from build123d import *

# Parameters (mm, degrees)
SKETCH1_R           = 20
SKETCH1_R_2         = 2.5
BOSS_EXTRUDE1_DEPTH = 10
CUT_EXTRUDE1_DEPTH  = 30
FILLET1_R           = 6
CUT_EXTRUDE2_DEPTH  = 4
CUT_EXTRUDE3_DEPTH  = 6
SKETCH5_R           = 3.75
CUT_EXTRUDE4_DEPTH  = 3
CUT_EXTRUDE5_DEPTH  = 5
CUT_EXTRUDE6_DEPTH  = 7


with BuildPart() as part:
    # Sketch1 → Boss-Extrude1 (new body)
    with BuildSketch(Plane.XY):
        with BuildLine():
            Line((0, 5), (0, 40))
            ThreePointArc((0, 40), (-2.928932188, 47.071067812), (-10, 50))
            Line((-10, 50), (-20, 50))
            ThreePointArc((-20, 50), (-23.535533906, 51.464466094), (-25, 55))
            Line((-25, 55), (-25, 95))
            ThreePointArc((-25, 95), (-23.535533906, 98.535533906), (-20, 100))
            Line((-20, 100), (25, 100))
            ThreePointArc((25, 100), (28.535533906, 98.535533906), (30, 95))
            Line((30, 95), (30, 90))
            ThreePointArc((30, 90), (31.464466094, 86.464466094), (35, 85))
            Line((35, 85), (45, 85))
            ThreePointArc((45, 85), (48.535533906, 86.464466094), (50, 90))
            Line((50, 90), (50, 95))
            ThreePointArc((50, 95), (51.464466094, 98.535533906), (55, 100))
            Line((55, 100), (80, 100))
            ThreePointArc((80, 100), (83.535533906, 98.535533906), (85, 95))
            Line((85, 95), (85, 36))
            ThreePointArc((85, 36), (83.242640687, 31.757359313), (79, 30))
            ThreePointArc((79, 30), (58.114182378, 26.808820785), (40.36, 15.355))
            Line((40.36, 15.355), (26.706048875, 1.749781342))
            ThreePointArc((26.706048875, 1.749781342), (24.762144416, 0.4546726), (22.470999719, 0))
            Line((22.470999719, 0), (5, 0))
            ThreePointArc((5, 0), (1.464466094, 1.464466094), (0, 5))
        make_face()
        with Locations((40, 50)):
            Circle(SKETCH1_R, mode=Mode.SUBTRACT)
        with Locations((10, 5)):
            Circle(SKETCH1_R_2, mode=Mode.SUBTRACT)
        with Locations((10, 40)):
            Circle(SKETCH1_R_2, mode=Mode.SUBTRACT)
        with Locations((15, 50)):
            Circle(SKETCH1_R_2, mode=Mode.SUBTRACT)
        with Locations((-20, 55)):
            Circle(SKETCH1_R_2, mode=Mode.SUBTRACT)
        with Locations((-20, 90)):
            Circle(SKETCH1_R_2, mode=Mode.SUBTRACT)
        with Locations((20, 95)):
            Circle(SKETCH1_R_2, mode=Mode.SUBTRACT)
        with Locations((20, 76.86)):
            Circle(SKETCH1_R_2, mode=Mode.SUBTRACT)
        with Locations((60, 77.99)):
            Circle(SKETCH1_R_2, mode=Mode.SUBTRACT)
        with Locations((60, 95)):
            Circle(SKETCH1_R_2, mode=Mode.SUBTRACT)
        with Locations((80, 90)):
            Circle(SKETCH1_R_2, mode=Mode.SUBTRACT)
        with Locations((80, 55)):
            Circle(SKETCH1_R_2, mode=Mode.SUBTRACT)
        with Locations((65, 50)):
            Circle(SKETCH1_R_2, mode=Mode.SUBTRACT)
    extrude(amount=BOSS_EXTRUDE1_DEPTH)

    # Sketch2 → Cut-Extrude1 (cut)
    with BuildSketch(Plane(origin=(0, 100, 0), x_dir=(1, 0, 0), z_dir=(0, 1, 0))):
        Polygon((55, -10), (85, -5.7143), (85, -10), align=None)
    extrude(amount=-CUT_EXTRUDE1_DEPTH, mode=Mode.SUBTRACT)

    # Fillet1
    fillet1_edges = [part.edges().sort_by_distance(p)[0] for p in [
        (85, 70, 7.85715),
    ]]
    fillet(fillet1_edges, radius=FILLET1_R)

    # Sketch3 → Cut-Extrude2 (cut)
    with BuildSketch(Plane.XY.offset(10)):
        with BuildLine():
            Line((76.5, 61), (76.5, 39))
            ThreePointArc((76.5, 39), (75.328427125, 36.171572875), (72.5, 35))
            Line((72.5, 35), (68, 35))
            ThreePointArc((68, 35), (59.758366163, 33.845718429), (52.150943396, 30.471698113))
            ThreePointArc((52.150943396, 30.471698113), (40, 27), (27.849056604, 30.471698113))
            ThreePointArc((27.849056604, 30.471698113), (20.241633837, 33.845718429), (12, 35))
            Line((12, 35), (7.5, 35))
            ThreePointArc((7.5, 35), (4.671572875, 36.171572875), (3.5, 39))
            Line((3.5, 39), (3.5, 61))
            ThreePointArc((3.5, 61), (4.671572875, 63.828427125), (7.5, 65))
            Line((7.5, 65), (12, 65))
            ThreePointArc((12, 65), (20.241633837, 66.154281571), (27.849056604, 69.528301887))
            ThreePointArc((27.849056604, 69.528301887), (40, 73), (52.150943396, 69.528301887))
            ThreePointArc((52.150943396, 69.528301887), (59.758366163, 66.154281571), (68, 65))
            Line((68, 65), (72.5, 65))
            ThreePointArc((72.5, 65), (75.328427125, 63.828427125), (76.5, 61))
        make_face()
    extrude(amount=-CUT_EXTRUDE2_DEPTH, mode=Mode.SUBTRACT)

    # Sketch4 → Cut-Extrude3 (cut)
    with BuildSketch(Plane.XY.offset(10)):
        with BuildLine():
            Line((-15, 66), (-15, 89))
            ThreePointArc((-15, 89), (-13.242640687, 93.242640687), (-9, 95))
            Line((-9, 95), (9, 95))
            ThreePointArc((9, 95), (13.242640687, 93.242640687), (15, 89))
            Line((15, 89), (15, 87.10469))
            ThreePointArc((15, 87.10469), (14.661769972, 85.118648515), (13.685213073, 83.356519985))
            Line((13.685213073, 83.356519985), (-3.198536927, 62.251829985))
            ThreePointArc((-3.198536927, 62.251829985), (-5.284617461, 60.592180657), (-7.88375, 60))
            Line((-7.88375, 60), (-9, 60))
            ThreePointArc((-9, 60), (-13.242640687, 61.757359313), (-15, 66))
        make_face()
        with BuildLine():
            Line((5, 23.8912), (5, 16))
            ThreePointArc((5, 16), (6.757359313, 11.757359313), (11, 10))
            Line((11, 10), (22.83171, 10))
            ThreePointArc((22.83171, 10), (24.870928608, 10.357164944), (26.667368083, 11.386137511))
            Line((26.667368083, 11.386137511), (40, 22.47))
            ThreePointArc((40, 22.47), (30.130642928, 23.984324498), (21.304906792, 28.653775146))
            ThreePointArc((21.304906792, 28.653775146), (19.582266385, 29.573428915), (17.65554, 29.8912))
            Line((17.65554, 29.8912), (11, 29.8912))
            ThreePointArc((11, 29.8912), (6.757359313, 28.133840687), (5, 23.8912))
        make_face()
    extrude(amount=-CUT_EXTRUDE3_DEPTH, mode=Mode.SUBTRACT)

    # Sketch5 → Cut-Extrude4 (cut)
    with BuildSketch(Plane(origin=(0, 0, 0), x_dir=(-1, 0, 0), z_dir=(0, 0, -1))):
        with Locations((-65, 50)):
            Circle(SKETCH5_R)
        with Locations((-15, 50)):
            Circle(SKETCH5_R)
    extrude(amount=-CUT_EXTRUDE4_DEPTH, mode=Mode.SUBTRACT)

    # Sketch6 → Cut-Extrude5 (cut)
    with BuildSketch(Plane(origin=(0, 0, 0), x_dir=(-1, 0, 0), z_dir=(0, 0, -1))):
        Polygon((-56.824573519, 95), (-58.41228676, 97.75), (-61.58771324, 97.75), (-63.175426481, 95), (-61.58771324, 92.25), (-58.41228676, 92.25), align=None)
        Polygon((-56.824573519, 77.99), (-58.41228676, 80.74), (-61.58771324, 80.74), (-63.175426481, 77.99), (-61.58771324, 75.24), (-58.41228676, 75.24), align=None)
        Polygon((-16.824573519, 76.86), (-18.41228676, 79.61), (-21.58771324, 79.61), (-23.175426481, 76.86), (-21.58771324, 74.11), (-18.41228676, 74.11), align=None)
        Polygon((-16.824573519, 95), (-18.41228676, 97.75), (-21.58771324, 97.75), (-23.175426481, 95), (-21.58771324, 92.25), (-18.41228676, 92.25), align=None)
    extrude(amount=-CUT_EXTRUDE5_DEPTH, mode=Mode.SUBTRACT)

    # Sketch7 → Cut-Extrude6 (cut)
    with BuildSketch(Plane.XY.offset(10)):
        Polygon((-17.25, 91.58771324), (-20, 93.175426481), (-22.75, 91.58771324), (-22.75, 88.41228676), (-20, 86.824573519), (-17.25, 88.41228676), align=None)
        Polygon((-17.25, 56.58771324), (-20, 58.175426481), (-22.75, 56.58771324), (-22.75, 53.41228676), (-20, 51.824573519), (-17.25, 53.41228676), align=None)
        Polygon((82.75, 91.58771324), (80, 93.175426481), (77.25, 91.58771324), (77.25, 88.41228676), (80, 86.824573519), (82.75, 88.41228676), align=None)
        Polygon((82.75, 56.58771324), (80, 58.175426481), (77.25, 56.58771324), (77.25, 53.41228676), (80, 51.824573519), (82.75, 53.41228676), align=None)
        Polygon((13.175426481, 40), (11.58771324, 42.75), (8.41228676, 42.75), (6.824573519, 40), (8.41228676, 37.25), (11.58771324, 37.25), align=None)
        Polygon((13.175426481, 5), (11.58771324, 7.75), (8.41228676, 7.75), (6.824573519, 5), (8.41228676, 2.25), (11.58771324, 2.25), align=None)
    extrude(amount=-CUT_EXTRUDE6_DEPTH, mode=Mode.SUBTRACT)


solid = part.part
Input: part model. Units: mm. Frame: model coordinates. A direction names the side the tool comes from. Give positions to 0.01 mm unless a question says otherwise; leave off trailing zeros. Write each loop counter-clockwise with the first axis right and the second up, starting at its lowest first coordinate (ties: lowest second). Pieces come first, ordered by that corner, then holes.
Q1. Pull-direction query (X, two-part tool) for faces 1 (the face through (12.37, 38.606, 4.521)), 2 (the face through (14, 0, 5)), 3 (the face through (85, 59, 4)); classes: pulls with the +X half, pulls with the -X half, needs draft (parallel to the pull), parting line crosses it, or undercut.
Q2. Set-up query: faces 4 (the face through (83.289, 68.196, 7.887)), 5 (the face through (78.64, 57.39, 6.55)), 6 (the face through (60, 92.25, 2)). Return all of +Z, -Z, +X, -X, +Y, -Y with unobstructed straight access to the full face (end or side cutting, diameter ignored); none if empty.
Q3. First-contact query: P1, Ø3, axis at y = 18.5, z = 8, coming from the -X side; P2, Ø1, axis at x = 60, z = 2.5, coming from the -Y side; P3, Ø4, axis at y = 47, z = 1.5, coming from the -X side. Flat tips, straight axial feed; report the tip coordinate or a pass-through.
Q4. Material intervals for probe 1 along Y at (x, z) = (-20, 1.55); probe 2 along Y at (x, z) = (80, 1.25); probe 3 along Y at (x, z) = (60, 8.45), sorted ascending.
Q5. Section A-A, the plane x = 46.5. Output: boundary loops of the cut face in (y, z).
Filled in:
1. face 1: undercut
1. face 2: needs draft
1. face 3: pulls with the +X half
2. face 4: +Z, +X, +Y
2. face 5: +Z
2. face 6: -Z
3. P1: stops at x = 0
3. P2: stops at y = 27.31
3. P3: stops at x = -5.64
4. probe 1: y = 50 to 52.5, 57.5 to 87.5, 92.5 to 100
4. probe 2: y = 30.08 to 52.5, 57.5 to 87.5, 92.5 to 100
4. probe 3: y = 27.48 to 33.91, 66.09 to 75.49, 80.49 to 92.5, 97.5 to 100
5. outline: (20.57, 0) - (31.09, 0) - (31.09, 6) - (27.94, 6) - (27.94, 10) - (20.57, 10) - close; (68.91, 0) - (85.23, 0) - (85.23, 10) - (72.06, 10) - (72.06, 6) - (68.91, 6) - close
